```python
from build123d import *

# Parameters (mm, degrees)
F0_W     = 50.8
F0_H     = 50.8
F1_DEPTH = 12.7
F2_W     = 12.7
F2_H     = 50.8
F3_DEPTH = 38.1
F5_D     = 12.7


with BuildPart() as f1:
    # F0 (on Top) → F1 (new body)
    with BuildSketch(Plane.XY):
        with Locations((0.405492, -2.999011)):
            Rectangle(F0_W, F0_H)
    extrude(amount=F1_DEPTH)

    # F2 (on Top) → F3 (join)
    with BuildSketch(Plane.XY):
        with Locations((-18.677441, -2.73966)):
            Rectangle(F2_W, F2_H)
    extrude(amount=F3_DEPTH)

    # F5 (through all)
    with Locations(Plane(origin=(-25.027441, 0, 0), x_dir=(0, -1, 0), z_dir=(-1, 0, 0))):
        with Locations((0, 21.290614)):
            Hole(F5_D / 2)


solid = f1.part
```
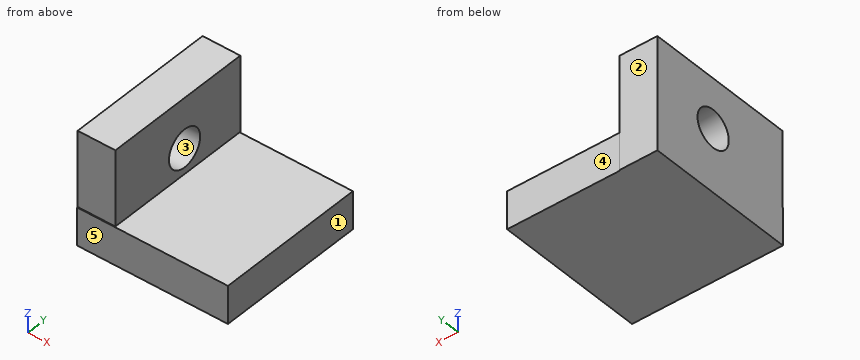
Read the model definition and answer for the solid it produces. Units are mm, in the model's axes. Face numbers are marked on the shaded views. A direction names the side the tool comes from. Round coordinates to 2 decimals unless told otherwise and drop trailing zeros. Write each loop counter-clockwise with the first axis right and the second up, starting at its lowest first coordinate (ties: lowest second). Pieces come first, ordered by that corner, then holes. Notation, with made-up numbers: (45.5, 77) - (54.5, 77) arc R20 ccw to (54.5, 115) - close; hole circle Ø1 at (74.25, 33.5). An arc over 180 degrees is marked (long way). One line per item, written item: value.
Q1. Find section C-C (y = 10). Determine the outline of the cut face in (x, z).
The answers:
outline: (-25.03, 0) - (25.81, 0) - (25.81, 12.7) - (-12.33, 12.7) - (-12.33, 38.1) - (-25.03, 38.1) - close
Q2. For a pull along Y with two mould halves and no side action, classify the marked faces 1, 2 and 3 as pulls with the +Y half, pulls with the -Y half, needs draft (parallel to the pull), parting line crosses it, or undercut.
The answers:
face 1: needs draft
face 2: pulls with the +Y half
face 3: undercut
Q3. Find section B-B (z = 23). Determine the outline of the cut face in (x, y).
The answers:
outline: (-25.03, -28.14) - (-12.33, -28.14) - (-12.33, -6.12) - (-25.03, -6.12) - close; (-25.03, 6.12) - (-12.33, 6.12) - (-12.33, 22.66) - (-25.03, 22.66) - close
Q4. Find section D-D (z = 30). Determine the outline of the cut face in (x, y).
The answers:
outline: (-25.03, -28.14) - (-12.33, -28.14) - (-12.33, 22.66) - (-25.03, 22.66) - close
Q5. Straight lines are drawn through the part: line 1 (Z direction, x = -16.5, y = 0); line 2 (X direction, y = 16.5, z = 23); line 3 (Z direction, x = -8.5, y = 5.5). For each, find the intervals that lie inside material, in ascending order. Write a range as from..to.
The answers:
line 1: z = 0..14.94, 27.64..38.1
line 2: x = -25.03..-12.33
line 3: z = 0..12.7
Q6. Find section A-A (y = 0). Determine the outline of the cut face in (x, z), and give its area (3 significant figures).
The answers:
outline: (-25.03, 0) - (25.81, 0) - (25.81, 12.7) - (-12.33, 12.7) - (-12.33, 14.94) - (-25.03, 14.94) - close; (-25.03, 27.64) - (-12.33, 27.64) - (-12.33, 38.1) - (-25.03, 38.1) - close
area: 807 mm2
Q7. Which of the six approach directions +Z, -Z, +X, -X, +Y, -Y give full straight-line access (tool end or side, diameter ignored) to the marked faces 4 and 5?
The answers:
face 4: +Z, -Z, +X, +Y
face 5: +Z, -Z, +X, -X, -Y
Q8. Each of these flat-tipped pins is pushed along its axis until it touches: P1, Ø3, axis at x = -19, z = 30, coming from the -Y side; P2, Ø8, axis at y = 1, z = 17.5, coming from the +X side; P3, Ø3, axis at x = 8, y = -10, coming from the -Z side; P4, Ø10, axis at x = 5.5, z = 4, coming from the +Y side. Where does it stop, or does it pass through?
The answers:
P1: stops at y = -28.14
P2: stops at x = -12.33
P3: stops at z = 0
P4: stops at y = 22.4
